Work out the finished part from the listing and answer in its coordinate system (mm). A direction names the side the tool comes from. Coordinates: 2 decimals unless noted, no trailing zeros. Order: outer loops, then holes, each group sorted by start corner. A loop starts at its lowest first (then second) coordinate and runs counter-clockwise, first axis right, second up. Notation, with made-up numbers: M 59,50.5 L 92,50.5 A17 ccw 92,80.5 Z; hole C 35.5,1 d8. An arc over 180 degrees is marked long. Use a Markdown table: item, result.
from build123d import *

# Parameters (mm, degrees)
F1_R     = 3.25
F3_DEPTH = 10
F0_R     = 34.5
F4_DEPTH = 36
F2_R     = 4.5
F5_DEPTH = 43
F6_R     = 5
F7_R     = 3.25
F8_DEPTH = 10


with BuildPart() as f3:
    # F1 (on Top) → F3 (new body)
    with BuildSketch(Plane.XY):
        Circle(F1_R)
    extrude(amount=F3_DEPTH)

    # F0 (on Top) → F4 (join)
    with BuildSketch(Plane.XY):
        Circle(F0_R)
    extrude(amount=F4_DEPTH)

    # F2 (on Top) → F5 (join)
    with BuildSketch(Plane.XY):
        Circle(F2_R)
    extrude(amount=F5_DEPTH)

    # F6
    f6_edges = [f3.edges().sort_by_distance(p)[0] for p in [
        (-34.5, 0, 36),
    ]]
    fillet(f6_edges, radius=F6_R)

    # F7 (on face) → F8 (cut)
    with BuildSketch(Plane.XY.offset(43)):
        Circle(F7_R)
    extrude(amount=-F8_DEPTH, mode=Mode.SUBTRACT)


solid = f3.part
1. Section D-D on z = 18 is taken. Determine the outline of the cut face in (x, y).
Answers below:
| item | result |
|---|---|
| outline | C 0,0 d69 |
2. For a pull along Y with two mould halves and no side action, classify faces 3 (the face through (-0.59, 4.46, 39.45)), 4 (the face through (0, 0, 0)), 5 (the face through (-2.579, -1.978, 38.07)) as +Y half, -Y half, draft (parallel to the pull), parting line (faces both ways), or undercut.
Answers below:
| item | result |
|---|---|
| face 3 | parting line |
| face 4 | draft |
| face 5 | undercut |
3. Flat-ended cylindrical pins translate along their axes: P1, Ø4, axis at x = -8.5, z = 29, coming from the -Y side; P2, Ø3, axis at x = 9, y = -15.5, coming from the +Z side; P3, Ø2, axis at y = -13, z = 9, coming from the -X side. Find the tip coordinate at first contact, or state that the pin passes through.
Answers below:
| item | result |
|---|---|
| P1 | y = -33.88 |
| P2 | z = 36 |
| P3 | x = -32.35 |
4. Find the intervals of material crossed by probe 1 along Y at (x, z) = (0, 38); probe 2 along Z at (x, y) = (16.5, -12.5); probe 3 along X at (y, z) = (10, 26.5), in increasing order.
Answers below:
| item | result |
|---|---|
| probe 1 | -4.5 to -3.25, 3.25 to 4.5 |
| probe 2 | 0 to 36 |
| probe 3 | -33.02 to 33.02 |
5. Section A-A on x = 0 is taken. Determine the outline of the cut face in (y, z), then the cut area to 3 significant figures.
Answers below:
| item | result |
|---|---|
| outline | M -34.5,0 L 34.5,0 L 34.5,31 A5 ccw 29.5,36 L 4.5,36 L 4.5,43 L 3.25,43 L 3.25,33 L -3.25,33 L -3.25,43 L -4.5,43 L -4.5,36 L -29.5,36 A5 ccw -34.5,31 Z |
| area | 2,470 mm² |
6. Section C-C on z = 39 is taken. Determine the outline of the cut face in (x, y).
Answers below:
| item | result |
|---|---|
| outline | C 0,0 d9; hole C 0,0 d6.5 |
7. For faces 1 (the face through (3, -2, 43)), 2 (the face through (0, 0, 33)), determine the directions among +Z, -Z, +X, -X, +Y, -Y from which every point of the face is accessible in a straight line to the end or side of a thin tool.
Answers below:
| item | result |
|---|---|
| face 1 | +Z, +X, -X, +Y, -Y |
| face 2 | +Z |
